Model file for the job. Use its own axes, mm. Coordinates: 2 decimals unless noted, no trailing zeros. Loops run counter-clockwise (first coordinate to the right, second up) from the corner with the lowest first, then second, coordinate; pieces in that order, holes last. Notation, with made-up numbers: M 75,-0.5 L 126,-0.5 A38 cw 126,38.5 Z; hole C 76,36 d7. An arc over 180 degrees is marked long. Write item = value, one per line. Start each with the question number.
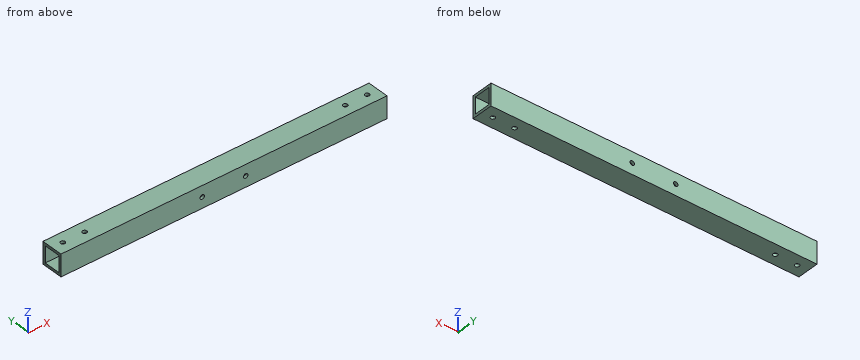
Autodesk Inventor part; units mm, degrees
ref_plane "YZ Plane" through (0, 0, 0) normal (1, 0, 0) x (0, 1, 0)
ref_plane "XZ Plane" through (0, 0, 0) normal (0, 1, 0) x (-1, 0, 0)
ref_plane "XY Plane" through (0, 0, 0) normal (0, 0, 1) x (1, 0, 0)
sketch "Sketch1" plane through (0, 0, 0) normal (1, 0, 0) x (0, 1, 0)
  line L0 (4.2484, 4.9473) -> (-21.1516, 4.9473)
  line L1 (-21.1516, 4.9473) -> (-21.1516, -20.4527)
  line L2 (-21.1516, -20.4527) -> (4.2484, -20.4527)
  line L3 (4.2484, -20.4527) -> (4.2484, 4.9473)
  line L4 (1.0734, 1.7723) -> (-17.9766, 1.7723)
  line L5 (-17.9766, 1.7723) -> (-17.9766, -17.2777)
  line L6 (-17.9766, -17.2777) -> (1.0734, -17.2777)
  line L7 (1.0734, -17.2777) -> (1.0734, 1.7723)
  point P0 (0, 0)
  dimension "d0" = 25.4
  dimension "d1" = 25.4
  dimension "d2" = 3.175
extrude "Extrusion1" add sketch "Sketch1" along normal blind 381
sketch "Sketch2" plane through (0, -21.1516, -20.4527) normal (0, 0, -1) x (-1, 0, 0)
  line L0 (0, 0) -> (0, 25.4) construction
  line L1 (0, 12.7) -> (-12.7, 12.7) construction
  line L2 (-12.7, 12.7) -> (-38.1, 12.7) construction
  line L3 (-381, 0) -> (-381, 25.4) construction
  line L4 (-381, 12.7) -> (-368.3, 12.7) construction
  line L5 (-368.3, 12.7) -> (-342.9, 12.7) construction
  circle A0 centre (-368.3, 12.7) radius 2.5797
  circle A1 centre (-342.9, 12.7) radius 2.5797
  circle A2 centre (-12.7, 12.7) radius 2.5797
  circle A3 centre (-38.1, 12.7) radius 2.5797
  point P0 (0, 21.1516)
  dimension "d5" = 12.7
  dimension "d6" = 25.4
  dimension "d7" = 12.7
  dimension "d8" = 25.4
  dimension "d9" = 5.1594
  dimension "d10" = 5.1594
  dimension "d11" = 5.1594
  dimension "d12" = 5.1594
extrude "Extrusion2" cut sketch "Sketch2" against normal blind 431.8
sketch "Sketch3" plane through (0, 4.2484, 4.9473) normal (0, 1, 0) x (1, 0, 0)
  line L0 (0, 25.4) -> (381, 25.4) construction
  line L1 (190.5, 25.4) -> (190.5, 12.7) construction
  line L2 (190.5, 25.4) -> (203.2, 25.4) construction
  line L3 (190.5, 12.7) -> (215.9, 12.7) construction
  line L4 (215.9, 12.7) -> (165.1, 12.7) construction
  circle A0 centre (165.1, 12.7) radius 2.5797
  circle A1 centre (215.9, 12.7) radius 2.5797
  point P0 (0, 4.9473)
  dimension "d15" = 12.7
  dimension "d16" = 90
  dimension "d17" = 25.4
  dimension "d18" = 50.8
  dimension "d19" = 5.1594
extrude "Extrusion3" cut sketch "Sketch3" against normal blind 77.7875
properties part number "17in 1x1 Beam"
Item 1: Cut at A-A (z = -14). Give the cut face in (x, y).
Item 2: Cut at B-B (x = 182.5). Give the cut face in (y, z), plus the area to 3 significant figures.
Item 3: Probe L1, parallel to Z at x = 303, y = -12.25; L2, parallel to X at y = -9.75, z = -18.5; L3, parallel to Y at x = 79, z = -6. List the from-to ranges inside material, lowest first.
Reported:
q1.outline = M 0,-21.15 L 381,-21.15 L 381,-17.98 L 0,-17.98 Z; M 0,1.07 L 381,1.07 L 381,4.25 L 0,4.25 Z
q2.outline = M -21.15,-20.45 L 4.25,-20.45 L 4.25,4.95 L -21.15,4.95 Z; hole M -17.98,-17.28 L 1.07,-17.28 L 1.07,1.77 L -17.98,1.77 Z
q2.area = 282 mm^2
q3.L1 = -20.45 to -17.28, 1.77 to 4.95
q3.L2 = 0 to 10.47, 14.93 to 35.87, 40.33 to 340.67, 345.13 to 366.07, 370.53 to 381
q3.L3 = -21.15 to -17.98, 1.07 to 4.25
